For this review, take the finished solid that the model builds, in its own axes (mm). Face numbers are marked on the shaded views. A direction names the side the tool comes from. Round coordinates to 2 decimals unless told otherwise and drop trailing zeros. Loops run counter-clockwise (first coordinate to the right, second up) from the corner with the lowest first, then second, coordinate; pieces in that order, holes last.
1. Consider section C-C on x = 28.5. State the section outline as (y, z) points.
2. Consider section A-A on z = 32.5. State the section outline as (x, y) points (3 decimals), then the cut area to 3 significant figures.
3. Draft analysis for pull direction Y (two halves, no side actions). For the marked faces 1, 2, 3 and 4, state which applies: released by +Y, released by -Y, zero draft, split by the parting line, or undercut.
4. Consider section B-B on y = 86. State the section outline as (x, z) points.
5. Tool access review of the marked faces 5 and 6: name each direction out of +Z, -Z, +X, -X, +Y, -Y from which nothing blocks a thin tool from reaching the whole face with its end or side.
6. To check wall thickness, follow line 1 along X through (y, z) = (27.5, 26.5); line 2 along Y through (x, z) = (40.5, 35); line 3 along X through (y, z) = (91, 20). State the ranges of each line that lie inside material, in increasing order.
7. Consider section D-D on y = 45. State the section outline as (x, z) points.
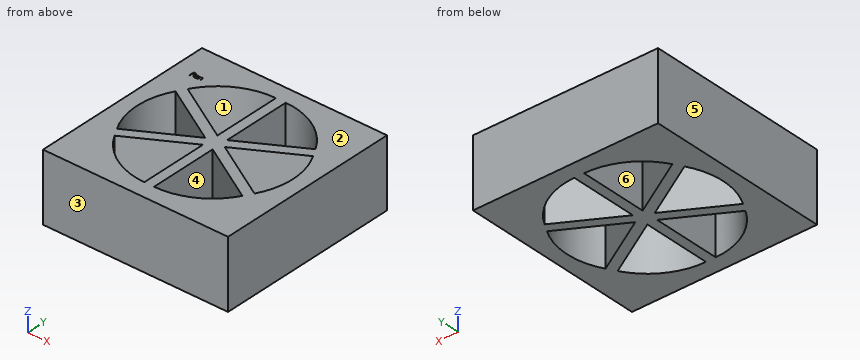
from build123d import *

# Parameters (mm, degrees)
SKETCH1_W           = 120.65
SKETCH1_H           = 120.65
BOSS_EXTRUDE1_DEPTH = 44.45
CUT_EXTRUDE1_DEPTH  = 3.175
CUT_EXTRUDE2_DEPTH  = 177.319731024


with BuildPart() as part:
    # Sketch1 → Boss-Extrude1 (new body)
    with BuildSketch(Plane.XY):
        with Locations((60.325, 60.325)):
            Rectangle(SKETCH1_W, SKETCH1_H)
    extrude(amount=BOSS_EXTRUDE1_DEPTH)

    # Sketch2 → Cut-Extrude1 (cut)
    # profile 1 of 3: a face of its own
    with BuildSketch(Plane.XY.offset(44.45)):
        Polygon((11.239986737, 101.279136985), (12.786781609, 101.279136985), (12.786781609, 100.953495959), (11.524922635, 100.953495959), (11.524922635, 99.976572882), (12.786781609, 99.976572882), (12.786781609, 99.650931857), (11.524922635, 99.650931857), (11.524922635, 98.104136985), (11.239986737, 98.104136985), align=None)
    # profile 2 of 3: a face of its own
    with BuildSketch(Plane.XY.offset(44.45)):
        with BuildLine():
            Line((15.636140583, 100.424329293), (15.636140583, 98.104136985))
            Line((15.636140583, 98.104136985), (15.351204686, 98.104136985))
            Line((15.351204686, 98.104136985), (15.351204686, 98.505464108))
            add(Edge.make_bspline(
                [(15.351204686, 98.505464108), (15.319074783, 98.469142477), (15.256372873, 98.398260356), (15.151651288, 98.305657242), (15.040645869, 98.22911405), (14.923895385, 98.167292341), (14.801505264, 98.120853833), (14.673746814, 98.087846389), (14.540567918, 98.066624838), (14.449624711, 98.064505733), (14.40353842, 98.063431857)],
                knots=[0, 0, 0, 0, 1.074387032, 2.096679803, 3.090159297, 4.057316773, 5.018401886, 5.985159533, 6.978961417, 8, 8, 8, 8], degree=3))
            add(Edge.make_bspline(
                [(14.40353842, 98.063431857), (14.362564633, 98.064544352), (14.281762512, 98.066738241), (14.16290042, 98.08375833), (14.048516737, 98.111091109), (13.938503374, 98.149101201), (13.833572214, 98.199520947), (13.732824841, 98.259883364), (13.636783184, 98.331766117), (13.546911145, 98.4139424), (13.464150688, 98.50320071), (13.391523676, 98.598401313), (13.330969097, 98.699132546), (13.280332309, 98.80411905), (13.241328482, 98.914169013), (13.214138114, 99.028901872), (13.197137852, 99.148181972), (13.19494487, 99.229407111), (13.193832891, 99.270593315)],
                knots=[0, 0, 0, 0, 1.033919861, 2.038935746, 3.024066025, 3.998881131, 4.97069526, 5.957263378, 6.95902576, 7.993208707, 9.027059324, 10.027763471, 11.009749337, 11.988697705, 12.965288445, 13.950418724, 14.960734635, 16, 16, 16, 16], degree=3))
            add(Edge.make_bspline(
                [(13.193832891, 99.270593315), (13.194969515, 99.310928246), (13.19721656, 99.390668229), (13.213956266, 99.507942476), (13.242105824, 99.620898327), (13.281609943, 99.729172126), (13.332266573, 99.832894886), (13.393887052, 99.932139965), (13.46647583, 100.027180776), (13.550161942, 100.115782532), (13.640817055, 100.197625518), (13.737798546, 100.268753723), (13.838693952, 100.330182579), (13.945068254, 100.378853947), (14.055346985, 100.418232206), (14.170511896, 100.445476398), (14.290083828, 100.461530397), (14.371264489, 100.46385519), (14.412442667, 100.465034421)],
                knots=[0, 0, 0, 0, 1.020392517, 2.01726096, 2.990465484, 3.961182959, 4.928053699, 5.906110375, 6.912531644, 7.948652711, 8.985773172, 9.998621852, 10.987621588, 11.969261332, 12.953316658, 13.946091881, 14.958173133, 16, 16, 16, 16], degree=3))
            add(Edge.make_bspline(
                [(14.412442667, 100.465034421), (14.459795396, 100.463730175), (14.552651863, 100.46117261), (14.688476557, 100.439888564), (14.816968334, 100.403930812), (14.939119067, 100.355019939), (15.054490118, 100.290024306), (15.161989254, 100.20803677), (15.262741514, 100.109574407), (15.321143636, 100.033945504), (15.351204686, 99.995017394)],
                knots=[0, 0, 0, 0, 1.038897134, 2.037228247, 3.008116434, 3.962042015, 4.918381754, 5.904844433, 6.921570401, 8, 8, 8, 8], degree=3))
            Line((15.351204686, 99.995017394), (15.351204686, 100.424329293))
            Line((15.351204686, 100.424329293), (15.636140583, 100.424329293))
        make_face()
        with BuildLine():
            add(Edge.make_bspline(
                [(14.416258772, 100.180098523), (14.374607909, 100.178616581), (14.292395729, 100.175691461), (14.171705813, 100.152855505), (14.056214359, 100.114860194), (13.946498991, 100.062897327), (13.844292823, 99.997556973), (13.752949279, 99.918525432), (13.671721257, 99.827958998), (13.603405903, 99.726266369), (13.547715952, 99.617247672), (13.508557288, 99.503288361), (13.482731613, 99.386443845), (13.480093169, 99.307193409), (13.478768789, 99.267413227)],
                knots=[0, 0, 0, 0, 1.031046209, 2.035121221, 3.029706178, 4.034933723, 5.034054252, 6.02443088, 7.017295772, 8.038157696, 9.050218397, 10.03989886, 11.016116709, 12, 12, 12, 12], degree=3))
            add(Edge.make_bspline(
                [(13.478768789, 99.267413227), (13.480460513, 99.227870773), (13.483837331, 99.148940857), (13.508104033, 99.031937048), (13.548816489, 98.917950881), (13.604371789, 98.807949837), (13.673937513, 98.705819975), (13.754572219, 98.613527149), (13.847055689, 98.534161594), (13.94949707, 98.467724652), (14.058905729, 98.414055794), (14.173962224, 98.376712678), (14.292503696, 98.352602834), (14.373105456, 98.34978663), (14.413714702, 98.348367754)],
                knots=[0, 0, 0, 0, 0.979072187, 1.954306742, 2.945804271, 3.96968567, 4.997920485, 5.998718438, 6.996577872, 8.005894225, 9.015743152, 10.005417472, 10.995077863, 12, 12, 12, 12], degree=3))
            add(Edge.make_bspline(
                [(14.413714702, 98.348367754), (14.454941172, 98.349873579), (14.536936533, 98.352868514), (14.657984504, 98.375802233), (14.775454934, 98.4136925), (14.887747634, 98.46621528), (14.992355839, 98.531309452), (15.086243199, 98.607515885), (15.165632685, 98.696146631), (15.232935981, 98.793552413), (15.285709394, 98.90033401), (15.324150534, 99.014030026), (15.346878006, 99.134644419), (15.349742517, 99.217070981), (15.351204686, 99.259144998)],
                knots=[0, 0, 0, 0, 1.01762866, 2.023962475, 3.030623092, 4.058876274, 5.077231937, 6.066672613, 7.034107872, 8.005628644, 8.981990164, 9.965428785, 10.961468474, 12, 12, 12, 12], degree=3))
            add(Edge.make_bspline(
                [(15.351204686, 99.259144998), (15.350334141, 99.291201458), (15.348620632, 99.354298717), (15.335530044, 99.446942965), (15.314706646, 99.535601417), (15.285364049, 99.620367285), (15.246818384, 99.700771906), (15.200329339, 99.777392602), (15.145079395, 99.849830873), (15.08195795, 99.91708923), (15.01286523, 99.978436092), (14.939754468, 100.033195082), (14.861759462, 100.078179183), (14.780191864, 100.115409479), (14.694910154, 100.145035994), (14.605220377, 100.164800545), (14.512075868, 100.178371693), (14.448534089, 100.179516853), (14.416258772, 100.180098523)],
                knots=[0, 0, 0, 0, 1.050140795, 2.067009409, 3.05949893, 4.030605086, 5.00011959, 5.97591094, 6.962425594, 7.979863591, 8.993523472, 9.986985069, 10.967611495, 11.937549037, 12.921786183, 13.919465291, 14.943216303, 16, 16, 16, 16], degree=3))
        make_face(mode=Mode.SUBTRACT)
    # profile 3 of 3: a face of its own
    with BuildSketch(Plane.XY.offset(44.45)):
        with BuildLine():
            Line((16.287422635, 100.424329293), (16.572358532, 100.424329293))
            Line((16.572358532, 100.424329293), (16.572358532, 100.005829693))
            add(Edge.make_bspline(
                [(16.572358532, 100.005829693), (16.602781958, 100.04378702), (16.661819678, 100.117444538), (16.760139752, 100.214255345), (16.864047433, 100.294034228), (16.972906393, 100.357628384), (17.08686441, 100.405567823), (17.20522684, 100.440189775), (17.328702324, 100.460949584), (17.412671491, 100.46366215), (17.455151, 100.465034421)],
                knots=[0, 0, 0, 0, 1.12780773, 2.188550248, 3.19190651, 4.159438251, 5.104880172, 6.052711206, 7.014878035, 8, 8, 8, 8], degree=3))
            add(Edge.make_bspline(
                [(17.455151, 100.465034421), (17.498086647, 100.463451279), (17.582122064, 100.460352689), (17.704475734, 100.435844691), (17.818751598, 100.393984352), (17.924542195, 100.336641974), (18.019907596, 100.265334673), (18.103659425, 100.182260543), (18.1729318, 100.086705667), (18.219375122, 99.998056804), (18.249969102, 99.919417684), (18.269229866, 99.852065275), (18.285586542, 99.777028095), (18.29976677, 99.694532896), (18.309361722, 99.60400168), (18.316929372, 99.50580556), (18.322352902, 99.399976341), (18.322568082, 99.326782044), (18.322679045, 99.289037826)],
                knots=[0, 0, 0, 0, 1.235846778, 2.418850247, 3.575807741, 4.728682307, 5.871620074, 6.994088408, 8.11269785, 9.256955736, 9.865816715, 10.540099792, 11.271859618, 12.076849838, 12.949306005, 13.892391288, 14.913166135, 16, 16, 16, 16], degree=3))
            Line((18.322679045, 99.289037826), (18.322679045, 98.104136985))
            Line((18.322679045, 98.104136985), (18.037743147, 98.104136985))
            Line((18.037743147, 98.104136985), (18.037743147, 99.195543235))
            add(Edge.make_bspline(
                [(18.037743147, 99.195543235), (18.03756788, 99.227132167), (18.037232624, 99.287556418), (18.036175216, 99.374069747), (18.03362632, 99.452525428), (18.030044636, 99.522735897), (18.02480223, 99.584633735), (18.019338843, 99.638345007), (18.012657756, 99.683801521), (18.006704257, 99.71116556), (18.004034213, 99.723437866)],
                knots=[0, 0, 0, 0, 1.430800155, 2.736877192, 3.918605307, 4.986035426, 5.920637409, 6.731861385, 7.431261377, 8, 8, 8, 8], degree=3))
            add(Edge.make_bspline(
                [(18.004034213, 99.723437866), (17.994395338, 99.759461584), (17.975843486, 99.828796095), (17.930001944, 99.922843544), (17.872113366, 100.0028519), (17.801448888, 100.068326497), (17.718691084, 100.119281471), (17.624069604, 100.154636415), (17.518497552, 100.176749174), (17.444243933, 100.178950929), (17.405541625, 100.180098523)],
                knots=[0, 0, 0, 0, 1.084156227, 2.086665306, 3.027808233, 3.945421172, 4.874247719, 5.839848303, 6.874090471, 8, 8, 8, 8], degree=3))
            add(Edge.make_bspline(
                [(17.405541625, 100.180098523), (17.382620226, 100.179666719), (17.337259371, 100.17881219), (17.269994753, 100.170238512), (17.204749253, 100.156215485), (17.140868064, 100.137284649), (17.079628851, 100.111283876), (17.019064101, 100.081775091), (16.961454393, 100.04499207), (16.905571312, 100.00399772), (16.853580408, 99.958568725), (16.805203986, 99.910631205), (16.762080211, 99.859581193), (16.72301077, 99.806241241), (16.689284774, 99.749878788), (16.659845187, 99.691037595), (16.634866378, 99.629640218), (16.622454221, 99.587027126), (16.616243748, 99.565705495)],
                knots=[0, 0, 0, 0, 1.023777757, 2.026029729, 3.023749952, 4.003683103, 4.997618607, 5.993177895, 7.010360494, 8.046726602, 9.087585522, 10.09234134, 11.086953743, 12.070360549, 13.043493632, 14.017870808, 15.008233677, 16, 16, 16, 16], degree=3))
            add(Edge.make_bspline(
                [(16.616243748, 99.565705495), (16.612669924, 99.55005256), (16.604889896, 99.515976941), (16.596486869, 99.460056647), (16.588859997, 99.395368312), (16.58247647, 99.321987425), (16.578570842, 99.239657066), (16.574312354, 99.148728842), (16.572761991, 99.048840178), (16.572496784, 98.979297071), (16.572358532, 98.943044237)],
                knots=[0, 0, 0, 0, 0.615963638, 1.340920617, 2.168419149, 3.115676021, 4.16674242, 5.331190069, 6.6087489, 8, 8, 8, 8], degree=3))
            Line((16.572358532, 98.943044237), (16.572358532, 98.104136985))
            Line((16.572358532, 98.104136985), (16.287422635, 98.104136985))
            Line((16.287422635, 98.104136985), (16.287422635, 100.424329293))
        make_face()
    extrude(amount=-CUT_EXTRUDE1_DEPTH, mode=Mode.SUBTRACT)

    # Sketch3 → Cut-Extrude2 (cut, through all)
    with BuildSketch(Plane.XY.offset(44.45)):
        with BuildLine():
            Line((66.675, 60.325), (105.169829198, 82.55))
            ThreePointArc((105.169829198, 82.55), (111.125, 60.325), (105.169829198, 38.1))
            Line((105.169829198, 38.1), (66.675, 60.325))
        make_face()
        with BuildLine():
            Line((63.5, 54.825738686), (101.994829198, 32.600738686))
            ThreePointArc((101.994829198, 32.600738686), (85.725, 16.330909488), (63.5, 10.375738686))
            Line((63.5, 10.375738686), (63.5, 54.825738686))
        make_face()
        with BuildLine():
            Line((57.15, 54.825738686), (57.15, 10.375738686))
            ThreePointArc((57.15, 10.375738686), (34.925, 16.330909488), (18.655170802, 32.600738686))
            Line((18.655170802, 32.600738686), (57.15, 54.825738686))
        make_face()
        with BuildLine():
            Line((53.975, 60.325), (15.480170802, 38.1))
            ThreePointArc((15.480170802, 38.1), (9.525, 60.325), (15.480170802, 82.55))
            Line((15.480170802, 82.55), (53.975, 60.325))
        make_face()
        with BuildLine():
            Line((57.15, 65.824261314), (18.655170802, 88.049261314))
            ThreePointArc((18.655170802, 88.049261314), (34.925, 104.319090512), (57.15, 110.274261314))
            Line((57.15, 110.274261314), (57.15, 65.824261314))
        make_face()
        with BuildLine():
            Line((63.5, 65.824261314), (63.5, 110.274261314))
            ThreePointArc((63.5, 110.274261314), (85.725, 104.319090512), (101.994829198, 88.049261314))
            Line((101.994829198, 88.049261314), (63.5, 65.824261314))
        make_face()
    extrude(amount=-CUT_EXTRUDE2_DEPTH, mode=Mode.SUBTRACT)


solid = part.part
Resolved:
1. outline: (0, 0) - (20.84, 0) - (20.84, 44.45) - (0, 44.45) - close; (38.28, 0) - (45.62, 0) - (45.62, 44.45) - (38.28, 44.45) - close; (75.03, 0) - (82.37, 0) - (82.37, 44.45) - (75.03, 44.45) - close; (99.81, 0) - (120.65, 0) - (120.65, 44.45) - (99.81, 44.45) - close
2. outline: (0, 0) - (120.65, 0) - (120.65, 120.65) - (0, 120.65) - close; hole (15.48, 38.1) - (53.975, 60.325) - (15.48, 82.55) arc R44.45 ccw to start; hole (18.655, 32.601) arc R44.45 ccw to (57.15, 10.376) - (57.15, 54.826) - close; hole (18.655, 88.049) - (57.15, 65.824) - (57.15, 110.274) arc R44.45 ccw to start; hole (63.5, 10.376) arc R44.45 ccw to (101.995, 32.601) - (63.5, 54.826) - close; hole (63.5, 65.824) - (101.995, 88.049) arc R44.45 ccw to (63.5, 110.274) - close; hole (66.675, 60.325) - (105.17, 38.1) arc R44.45 ccw to (105.17, 82.55) - close
2. area: 8,350 mm2
3. face 1: undercut
3. face 2: zero draft
3. face 3: released by -Y
3. face 4: undercut
4. outline: (0, 0) - (22.2, 0) - (22.2, 44.45) - (0, 44.45) - close; (57.15, 0) - (63.5, 0) - (63.5, 44.45) - (57.15, 44.45) - close; (98.45, 0) - (120.65, 0) - (120.65, 44.45) - (98.45, 44.45) - close
5. face 5: +Z, -Z, -X, +Y, -Y
5. face 6: +Z, -Z
6. line 1: x = 0 to 22.09, 57.15 to 63.5, 98.56 to 120.65
6. line 2: y = 0 to 13.61, 45.21 to 52.55, 68.1 to 75.44, 107.04 to 120.65
6. line 3: x = 0 to 20.52, 57.15 to 63.5, 100.13 to 120.65
7. outline: (0, 0) - (12.25, 0) - (12.25, 44.45) - (0, 44.45) - close; (27.43, 0) - (40.13, 0) - (40.13, 44.45) - (27.43, 44.45) - close; (57.15, 0) - (63.5, 0) - (63.5, 44.45) - (57.15, 44.45) - close; (80.52, 0) - (93.22, 0) - (93.22, 44.45) - (80.52, 44.45) - close; (108.4, 0) - (120.65, 0) - (120.65, 44.45) - (108.4, 44.45) - close
